Here's how the part is built. I have some questions about the finished solid (model axes, mm). Round coordinates to 2 decimals unless told otherwise and drop trailing zeros. Write each loop counter-clockwise with the first axis right and the second up, starting at its lowest first coordinate (ties: lowest second). Pieces come first, ordered by that corner, then holes. Notation, with made-up numbers: (19.5, 5.5) -> (61.5, 5.5) arc R20 ccw to (61.5, 25.5) -> close; hole circle Ø5 at (-10.5, -14.75). An arc over 180 degrees is marked (long way). Put each result on its own line as item: value. Start each with the question number.
1) Will these pins go through, and if not, where does the flat tip stop? P1, Ø6, axis at y = -66, z = 1331.5, coming from the +X side; P2, Ø2, axis at y = 11.5, z = 1661.5, coming from the -X side; P3, Ø2, axis at x = 147, z = 980.5, coming from the +Y side; P4, Ø10, axis at x = 7, y = 174, coming from the -Z side.
2) I want a section at D-D, the plane x = 23. List the corners of the cut face in (y, z) for me, then the cut area to 3 significant figures.
3) I want a section at B-B, the plane y = 184. List the corners of the cut face in (x, z) for me.
4) I want a section at A-A, the plane x = -226.5. List the corners of the cut face in (y, z) for me, then the cut area to 3 significant figures.
5) If I drill on line 1 along Y through (x, z) = (-160, 1922.5); line 2 along X through (y, z) = (260, 160); line 3 along Y through (x, z) = (-37, 321), over which ranges is the centre line in solid material (lowest first)? Write a range as [from, to].
6) I want a section at C-C, the plane z = 248. List the corners of the cut face in (x, y) for me.
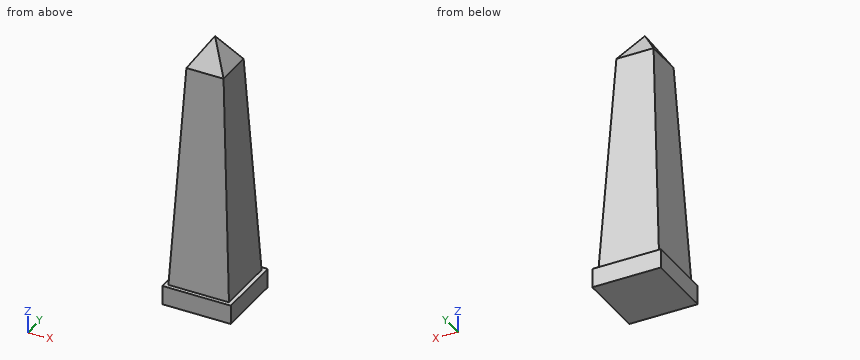
from build123d import *

# Parameters (mm, degrees)
F0_W     = 546.1
F0_H     = 546.1
F1_DEPTH = 152.4
F2_W     = 482.6
F2_H     = 482.6
F3_DEPTH = 1778
F3_TAPER = 3
F4_W     = 296.2379368695
F4_H     = 296.2379368695
F5_DEPTH = 241.3
F5_TAPER = 33


with BuildPart() as f1:
    # F0 (on Top) → F1 (new body)
    with BuildSketch(Plane.XY):
        with Locations((-51.5293031931, 57.3979665157)):
            Rectangle(F0_W, F0_H)
    extrude(amount=F1_DEPTH)

    # F2 (on face) → F3 (join)
    with BuildSketch(Plane.XY.offset(152.4)):
        with Locations((-51.5293031931, 57.3979665157)):
            Rectangle(F2_W, F2_H)
    extrude(amount=F3_DEPTH, taper=F3_TAPER)

    # F4 (on face) → F5 (join)
    with BuildSketch(Plane.XY.offset(1930.4)):
        with Locations((-51.5293031931, 57.3979665157)):
            Rectangle(F4_W, F4_H)
    extrude(amount=F5_DEPTH, taper=F5_TAPER)


solid = f1.part
Findings:
1. P1: stops at x = 128.13
1. P2: stops at x = -213.79
1. P3: stops at y = 255.34
1. P4: stops at z = 0
2. outline: (-215.65, 0) -> (330.45, 0) -> (330.45, 152.4) -> (298.7, 152.4) -> (205.52, 1930.4) -> (131.93, 2043.72) -> (-17.13, 2043.72) -> (-90.72, 1930.4) -> (-183.9, 152.4) -> (-215.65, 152.4) -> close
2. area: 801,000 mm2
3. outline: (-324.58, 0) -> (221.52, 0) -> (221.52, 152.4) -> (189.77, 152.4) -> (96.59, 1930.4) -> (75.07, 1963.53) -> (-178.13, 1963.53) -> (-199.65, 1930.4) -> (-292.83, 152.4) -> (-324.58, 152.4) -> close
4. outline: (-215.65, 0) -> (330.45, 0) -> (330.45, 152.4) -> (298.7, 152.4) -> (232.37, 1418.04) -> (-117.57, 1418.04) -> (-183.9, 152.4) -> (-215.65, 152.4) -> close
4. area: 610,000 mm2
5. line 1: y = [-91.14, 205.93]
5. line 2: x = [-292.43, 189.37]
5. line 3: y = [-175.07, 289.86]
6. outline: (-287.82, -178.89) -> (184.76, -178.89) -> (184.76, 293.69) -> (-287.82, 293.69) -> close
